The model under review builds one solid part; all positions refer to its coordinate system, in mm. Give positions to 0.01 mm unless a question says otherwise; leave off trailing zeros. Loops run counter-clockwise (first coordinate to the right, second up) from the corner with the lowest first, then second, coordinate; pieces in that order, holes last. Notation, with made-up numbers: (6.25, 75) - (14.25, 75) arc R24 ccw to (14.25, 97) - close; hole circle Ø7 at (29, 45.5). An arc over 180 degrees is marked (long way). Return JSON: item names as keys, results as strings. Group by question number.
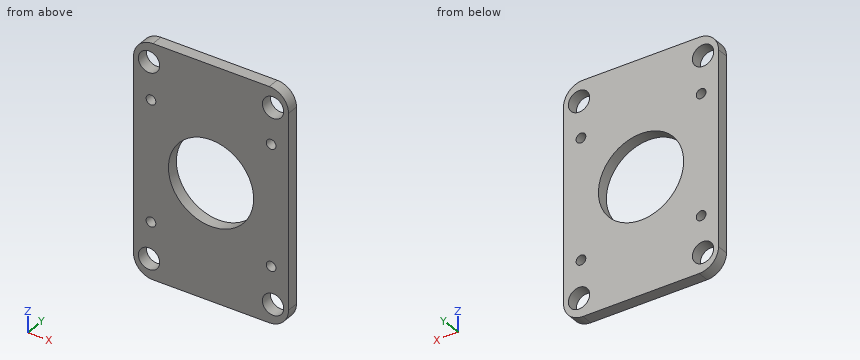
from build123d import *

# Parameters (mm, degrees)
SKETCH1_W           = 40
SKETCH1_H           = 60
SKETCH1_R           = 2.75
SKETCH1_R_2         = 1.25
SKETCH1_R_3         = 11
SKETCH1_R_4         = 4
BOSS_EXTRUDE1_DEPTH = 3
FILLET1_R           = 5


with BuildPart() as part:
    # Sketch1 → Boss-Extrude1 (new body)
    # profile 1 of 3: a face of its own
    with BuildSketch(Plane(origin=(0, 0, 0), x_dir=(1, 0, 0), z_dir=(0, 1, 0))):
        Rectangle(SKETCH1_W, SKETCH1_H)
        with Locations(Location((16, -25, 0), (0, 0, 270))):
            Circle(SKETCH1_R, mode=Mode.SUBTRACT)
        with Locations(Location((-16, -25, 0), (0, 0, 270))):
            Circle(SKETCH1_R, mode=Mode.SUBTRACT)
        with Locations(Location((16, 25, 0), (0, 0, 270))):
            Circle(SKETCH1_R, mode=Mode.SUBTRACT)
        with Locations(Location((-16, 25, 0), (0, 0, 270))):
            Circle(SKETCH1_R, mode=Mode.SUBTRACT)
        with Locations(Location((15.5, -15.5, 0), (0, 0, 270))):
            Circle(SKETCH1_R_2, mode=Mode.SUBTRACT)
        with Locations(Location((15.5, 15.5, 0), (0, 0, 270))):
            Circle(SKETCH1_R_2, mode=Mode.SUBTRACT)
        with Locations(Location((-15.5, 15.5, 0), (0, 0, 270))):
            Circle(SKETCH1_R_2, mode=Mode.SUBTRACT)
        with Locations(Location((-15.5, -15.5, 0), (0, 0, 270))):
            Circle(SKETCH1_R_2, mode=Mode.SUBTRACT)
        with Locations(Location((0, 0, 0), (0, 0, 270))):
            Circle(SKETCH1_R_3, mode=Mode.SUBTRACT)
        with Locations((0, 25)):
            Circle(SKETCH1_R_4, mode=Mode.SUBTRACT)
        with Locations((0, -25)):
            Circle(SKETCH1_R_4, mode=Mode.SUBTRACT)
    # profile 2 of 3: a face of its own
    with BuildSketch(Plane(origin=(0, 0, 0), x_dir=(1, 0, 0), z_dir=(0, 1, 0))):
        with Locations((0, 25)):
            Circle(SKETCH1_R_4)
    # profile 3 of 3: a face of its own
    with BuildSketch(Plane(origin=(0, 0, 0), x_dir=(1, 0, 0), z_dir=(0, 1, 0))):
        with Locations((0, -25)):
            Circle(SKETCH1_R_4)
    extrude(amount=BOSS_EXTRUDE1_DEPTH)

    # Fillet1
    fillet1_edges = [part.edges().sort_by_distance(p)[0] for p in [
        (20, 1.5, 30),
        (-20, 1.5, 30),
        (-20, 1.5, -30),
        (20, 1.5, -30),
    ]]
    fillet(fillet1_edges, radius=FILLET1_R)


solid = part.part
Item 1: For P1, Ø4.5, axis at x = -16, z = 25, coming from the +Y side; P2, Ø4, axis at x = -15.5, z = -15.5, coming from the -Y side, all flat-tipped, find the tip position at first contact; note any pin that passes through.
Item 2: Take a section at C-C (z = 15.5). State the section outline as (x, y) points, then the cut area to 3 significant figures.
Item 3: Take a section at B-B (x = 0). State the section outline as (y, z) points, then the cut area to 3 significant figures.
Item 4: Take a section at D-D (y = 1.2). State how many separate pieces and enclosed holes the cut face has, then the cut area to 3 significant figures.
Item 5: Take a section at A-A (z = 0). State the section outline as (x, y) points, then the cut area to 3 significant figures.
Item 6: For L1, parallel to X at y = 1.75, z = -15.5; L2, parallel to X at y = 2.1, z = 0; L3, parallel to Z at x = 17.5, y = 1.7, list the stretches that pass through material, from the lowest coordinate up. Write a range as from..to.
Check sheet entries:
{
 "1": {"P1": "passes through", "P2": "stops at y = 0"},
 "2": {"outline": "(-20, 0) - (-16.75, 0) - (-16.75, 3) - (-20, 3) - close; (-14.25, 0) - (14.25, 0) - (14.25, 3) - (-14.25, 3) - close; (16.75, 0) - (20, 0) - (20, 3) - (16.75, 3) - close", "area": "105 mm^2"},
 "3": {"outline": "(0, -30) - (3, -30) - (3, -11) - (0, -11) - close; (0, 11) - (3, 11) - (3, 30) - (0, 30) - close", "area": "114 mm^2"},
 "4": {"separate pieces": "1", "enclosed holes": "9", "area": "1,880 mm^2"},
 "5": {"outline": "(-20, 0) - (-11, 0) - (-11, 3) - (-20, 3) - close; (11, 0) - (20, 0) - (20, 3) - (11, 3) - close", "area": "54.0 mm^2"},
 "6": {"L1": "x = -20..-16.75, -14.25..14.25, 16.75..20", "L2": "x = -20..-11, 11..20", "L3": "z = -29.33..-27.3, -22.7..22.7, 27.3..29.33"}
}
